Here's how the part is built. I have some questions about the finished solid (model axes, mm). A direction names the side the tool comes from. Coordinates: 2 decimals unless noted, no trailing zeros. Write each loop counter-clockwise with the first axis right and the second up, starting at its lowest first coordinate (ties: lowest second). Pieces come first, ordered by that corner, then holes.
(1) Imagine slicing it at A-A, the plane x = 0. List the corners of the cut face in (y, z) for me (3 decimals).
(2) Imagine slicing it at C-C, the plane y = 208. List the corners of the cut face in (x, z) for me.
(3) Please list where these lines run through material, in increasing order: probe 1 along X at (y, z) = (221.5, 62); probe 2 along X at (y, z) = (213.5, 27); probe 3 along Z at (x, y) = (-73, 204).
(4) Thinking about a two-plate mould opening in X: for faces 5 (the flat face through (-108, 234, 0)), 6 (the conical face through (-2.2, 193.2, 99.9)), 7 (the conical face through (-2.563, 273.656, 116.535)), which applies, released by +X, released by -X, zero draft, split by the parting line, or undercut?
(5) For pin 1 Ø3 at (y, z) = (254, 32.5) entering from +X; pin 2 Ø1 at (y, z) = (208.5, 48) entering from +X; pin 3 Ø5 at (x, y) = (-15, 244) entering from +Z, each with a flat end and sliding along its axis, tell me the tip position at first contact or that it passes through.
(6) Imagine slicing it at B-B, the plane y = 230. List the corners of the cut face in (x, z) for me.
(7) Which directions (+Z, -Z, +X, -X, +Y, -Y) give clear straight access to the entire face, cutting with the end or side of a thin tool? Please do faces 1 (the conical face through (-2.565, 273.232, 116.619)), 2 (the conical face through (-2.14, 187.54, 97.42)), 3 (the conical face through (-2.288, 224.236, 104.024)), 4 (the conical face through (-2.519, 273.666, 114.548)).
```python
from build123d import *

# Parameters (mm, degrees)
RIB5_START          = -1.5875
RIB5_DEPTH          = 3.175
CIRPATTERN1_COUNT   = 4
BOSS_EXTRUDE1_REACH = 604.818
SKETCH4_R           = 50.8
SKETCH4_R_2         = 44.45
SKETCH4_3_R         = 44.45
CUT_EXTRUDE1_DEPTH  = 155.575
SKETCH16_R          = 47.625
SKETCH16_R_2        = 44.45
CUT_EXTRUDE8_DEPTH  = 165.1
BOSS_EXTRUDE2_START = 127
SKETCH10_R          = 53.975
SKETCH10_R_2        = 50.8
BOSS_EXTRUDE2_DEPTH = 127
RIB10_START         = -3.175
RIB10_DEPTH         = 3.175
SKETCH12_R          = 50.8
CUT_EXTRUDE4_DEPTH  = 9.525
SKETCH17_R          = 3.175
CUT_EXTRUDE9_DEPTH  = 3.175
SKETCH18_W          = 50.8
SKETCH18_H          = 130.175
SKETCH19_W          = 254
SKETCH19_H          = 114.3
CUT_EXTRUDE10_DEPTH = 326.542078986


with BuildPart() as part:
    # Sketch1 → Revolve-Thin1 (revolve)
    with BuildSketch(Plane.XY, mode=Mode.PRIVATE) as revolve_thin1_sk:
        Polygon((-104.775, 0), (-60.325, 0), (-158.75, 469.9), (-50.8, 469.9), (-50.8, 466.725), (-154.841065026, 466.725), (-56.416065026, -3.175), (-104.775, -3.175), align=None)
    revolve(revolve_thin1_sk.sketch.rotate(Axis((0, 0, 0), (0, 1, 0)), 270), axis=Axis((0, 0, 0), (0, 1, 0)))

    # Rib5: read off the stored shape, not the designer's step
    # Rib5 outline → Rib5 (add)
    with BuildSketch(Plane(origin=(0, 0, 0), x_dir=(0, 0, -1), z_dir=(1, 0, 0)).offset(RIB5_START)):
        with BuildLine():
            add(Edge.make_bspline(
                [(-60.304108235, -2e-09), (-60.337817831, 0.160880416), (-60.371527408, 0.321760839), (-62.968360223, 12.715265359), (-65.531376886, 24.947911788), (-71.07360722, 51.400397829), (-74.052795216, 65.620242821), (-77.031911205, 79.840102899)],
                knots=[1388.368707512, 1388.368707512, 1388.368707512, 1388.368707512, 1388.861829823, 1388.861829823, 1426.356632629, 1426.356632629, 1469.942363945, 1469.942363945, 1469.942363945, 1469.942363945], degree=3))
            Line((-77.031911205, 79.840102899), (-98.425, 0))
            Line((-98.425, 0), (-60.304108235, -2e-09))
        make_face()
    rib5 = extrude(amount=RIB5_DEPTH)

    # CirPattern1: Rib5 ×4 about axis
    cirpattern1_axis = Axis((0, 0, 0), (0, 1, 0))
    for i in range(1, CIRPATTERN1_COUNT):
        add(rib5.rotate(cirpattern1_axis, i * 360 / CIRPATTERN1_COUNT))

    # Sketch4 → Boss-Extrude1 (add, up to next)
    with BuildSketch(Plane(origin=(0, 41.317067623, 234.320734449), x_dir=(-1, 0, 0), z_dir=(0, 0.17364817766693072, 0.984807753012208)), mode=Mode.PRIVATE) as boss_extrude1_sk1:
        with Locations(Location((-89.350924276, -380.21116314, 0), (0, 0, 90))):
            Circle(SKETCH4_R)
        with Locations(Location((-89.350924276, -380.21116314, 0), (0, 0, 90))):
            Circle(SKETCH4_R_2, mode=Mode.SUBTRACT)
    boss_extrude1_tool1 = extrude(boss_extrude1_sk1.sketch, amount=-BOSS_EXTRUDE1_REACH, mode=Mode.PRIVATE) - part.part
    add(boss_extrude1_tool1.solids().sort_by_distance((89.350924, 464.365191, 159.725936))[0])

    # Sketch4<3> → Cut-Extrude1 (cut)
    with BuildSketch(Plane(origin=(0, 41.317067623, 234.320734449), x_dir=(-1, 0, 0), z_dir=(0, 0.17364817766693072, 0.984807753012208))):
        with Locations(Location((-89.350924276, -380.21116314, 0), (0, 0, 90))):
            Circle(SKETCH4_3_R)
    extrude(amount=-CUT_EXTRUDE1_DEPTH, mode=Mode.SUBTRACT)

    # Sketch16 → Cut-Extrude8 (cut)
    # profile 1 of 2: a face of its own
    with BuildSketch(Plane(origin=(0, 41.317067623, 234.320734449), x_dir=(1, 0, 0), z_dir=(0, 0.17364817766693058, 0.9848077530122081))):
        with Locations(Location((89.350924276, 380.21116314, 0), (0, 0, 270))):
            Circle(SKETCH16_R)
        with Locations((89.350924276, 380.21116314)):
            Circle(SKETCH16_R_2, mode=Mode.SUBTRACT)
    # profile 2 of 2: a face of its own
    with BuildSketch(Plane(origin=(0, 41.317067623, 234.320734449), x_dir=(1, 0, 0), z_dir=(0, 0.17364817766693058, 0.9848077530122081))):
        with Locations((89.350924276, 380.21116314)):
            Circle(SKETCH16_R_2)
    extrude(amount=-CUT_EXTRUDE8_DEPTH, mode=Mode.SUBTRACT)

    # Sketch10 → Boss-Extrude2 (add)
    with BuildSketch(Plane.XZ.offset(-466.725).offset(BOSS_EXTRUDE2_START)):
        with Locations(Location((0, 0, 0), (0, 0, 90))):
            Circle(SKETCH10_R)
        with Locations(Location((0, 0, 0), (0, 0, 270))):
            Circle(SKETCH10_R_2, mode=Mode.SUBTRACT)
    extrude(amount=-BOSS_EXTRUDE2_DEPTH)

    # Rib10: read off the stored shape, not the designer's step
    # Rib10 outline → Rib10 (add)
    with BuildSketch(Plane(origin=(41.275, 0, 0), x_dir=(0, 0, -1), z_dir=(1, 0, 0)).offset(RIB10_START)):
        with BuildLine():
            Line((-129.397511049, 371.475000111), (-34.780382402, 371.475))
            Line((-34.780382402, 371.475), (-34.780382402, 466.725))
            Line((-34.780382402, 466.725), (-150.08046179, 466.725000293))
            add(Edge.make_bspline(
                [(-129.397511049, 371.475000111), (-129.621022333, 372.498635621), (-129.844489601, 373.522280745), (-132.947477272, 387.73914033), (-135.819852259, 400.933914587), (-140.797597402, 423.849651078), (-142.905681683, 433.570024076), (-146.702544816, 451.101957641), (-148.392325081, 458.913301347), (-150.08046179, 466.725000293)],
                knots=[195.059408085, 195.059408085, 195.059408085, 195.059408085, 198.202667885, 198.202667885, 238.714059285, 238.714059285, 268.553076365, 268.553076365, 292.529147638, 292.529147638, 292.529147638, 292.529147638], degree=3))
        make_face()
    extrude(amount=RIB10_DEPTH)

    # Sketch12 → Cut-Extrude4 (cut)
    with BuildSketch(Plane(origin=(0, 41.317067623, 234.320734449), x_dir=(1, 0, 0), z_dir=(0, 0.17364817766693058, 0.9848077530122081))):
        with Locations(Location((89.350924276, 380.21116314, 0), (0, 0, 270))):
            Circle(SKETCH12_R)
    extrude(amount=-CUT_EXTRUDE4_DEPTH, mode=Mode.SUBTRACT)

    # Sketch17 → Cut-Extrude9 (cut)
    with BuildSketch(Plane.XZ.offset(3.175)):
        with Locations(Location((-62.861792847, 62.861792847, 0), (0, 0, 270))):
            Circle(SKETCH17_R)
        with Locations(Location((-34.020557137, 82.13289044, 0), (0, 0, 270))):
            Circle(SKETCH17_R)
        with Locations(Location((34.020557137, 82.13289044, 0), (0, 0, 270))):
            Circle(SKETCH17_R)
        with Locations(Location((62.861792847, 62.861792847, 0), (0, 0, 270))):
            Circle(SKETCH17_R)
        with Locations(Location((82.13289044, 34.020557137, 0), (0, 0, 270))):
            Circle(SKETCH17_R)
        with Locations(Location((82.13289044, -34.020557137, 0), (0, 0, 270))):
            Circle(SKETCH17_R)
        with Locations(Location((62.861792847, -62.861792847, 0), (0, 0, 270))):
            Circle(SKETCH17_R)
        with Locations(Location((34.020557137, -82.13289044, 0), (0, 0, 270))):
            Circle(SKETCH17_R)
        with Locations(Location((-34.020557137, -82.13289044, 0), (0, 0, 270))):
            Circle(SKETCH17_R)
        with Locations(Location((-62.861792847, -62.861792847, 0), (0, 0, 270))):
            Circle(SKETCH17_R)
        with Locations(Location((-82.13289044, -34.020557137, 0), (0, 0, 270))):
            Circle(SKETCH17_R)
        with Locations(Location((-82.13289044, 34.020557137, 0), (0, 0, 270))):
            Circle(SKETCH17_R)
    extrude(amount=-CUT_EXTRUDE9_DEPTH, mode=Mode.SUBTRACT)

    # Sketch18 → Cut-Revolve2 (revolve, cut)
    with BuildSketch(Plane.XY, mode=Mode.PRIVATE) as cut_revolve2_sk:
        Polygon((-114.410343119, 273.700908317), (-154.841065026, 466.725), (-56.416065026, 339.725), (-53.975, 339.725), (-50.8, 339.725), (-50.8, 469.9), (-158.75, 469.9), (-117.517905405, 273.05), (-116.48205131, 273.266969439), (-117.783867943, 279.482094012), (-116.748013848, 279.69906345), (-115.446197215, 273.483938878), align=None)
        Polygon((-56.416065026, -3.175), (-97.64815962, 193.675), (-98.684013716, 193.458030561), (-97.382197082, 187.242905988), (-98.418051178, 187.02593655), (-99.719867811, 193.241061122), (-100.755721907, 193.024091683), (-77.041088772, 79.805843168), (-98.425, 0), (-104.775, 0), (-104.775, -3.175), align=None)
        with Locations((-25.4, 404.8125)):
            Rectangle(SKETCH18_W, SKETCH18_H)
    revolve(cut_revolve2_sk.sketch.rotate(Axis((0, 0, 0), (0, 1, 0)), 270), axis=Axis((0, 0, 0), (0, 1, 0)), mode=Mode.SUBTRACT)


with BuildPart() as cut_revolve2_kept_piece:
    # of the separate pieces the step leaves, the one the design keeps (cut_revolve2_pieces_kept)
    add(part.part.solids().sort_by_distance((0, 193.024091683, -100.755721907))[0])

    # Sketch19 → Cut-Extrude10 (cut, through all)
    with BuildSketch(Plane.XY):
        with Locations((0, 233.254015281)):
            Rectangle(SKETCH19_W, SKETCH19_H)
    extrude(amount=-CUT_EXTRUDE10_DEPTH, mode=Mode.SUBTRACT)


solid = cut_revolve2_kept_piece.part
```
Recorded:
1. outline: (187.026, 98.418) - (187.243, 97.382) - (193.458, 98.684) - (193.675, 97.648) - (273.701, 114.41) - (273.484, 115.446) - (279.699, 116.748) - (279.482, 117.784) - (273.267, 116.482) - (273.05, 117.518) - (193.024, 100.756) - (193.241, 99.72) - close
2. outline: (-103.89, 0) - (-100.65, 0) arc R100.65 cw to (100.65, 0) - (103.89, 0) arc R103.89 ccw to start
3. probe 1: x = -86.86 to -82.85, 82.85 to 86.86
3. probe 2: x = -101.52 to -98.15, 98.15 to 101.52
3. probe 3: z = 68.07 to 72.74
4. face 5: zero draft
4. face 6: undercut
4. face 7: split by the parting line
5. pin 1: stops at x = 109.32
5. pin 2: stops at x = 92.54
5. pin 3: stops at z = 111.04
6. outline: (-108.5, 0) - (-105.26, 0) arc R105.26 cw to (105.26, 0) - (108.5, 0) arc R108.5 ccw to start
7. face 1: +Z
7. face 2: -Z
7. face 3: -Z, +Y
7. face 4: +Y
